The drawing under review shows one solid part. Ordinate dimensions are in mm from its lowest x, y, z. Coordinates: 2 decimals unless noted, no trailing zeros. Write each loop counter-clockwise with the first axis right and the second up, starting at its lowest first coordinate (ties: lowest second). Pieces come first, ordered by that corner, then holes.
Q1. Add section A-A, the plane z = 1188.5. Give the boundary of the cut face in (x, y).
Q2. Add section D-D, the plane x = 1858.5. Give the boundary of the cut face in (y, z) (1 decimal).
Q3. Clearance check with flat-ended pins moving along their axes: pin 1 Ø4 at (y, z) = (9, 1035) entering from -X; pin 2 Ø1.5 at (x, y) = (514, 6.5) entering from -Z; pin 3 Ø12 at (y, z) = (10, 1261.5) entering from -X (1 decimal). State where each tip first meets the part, or that it passes through.
Q4. Add section C-C, the plane z = 457. Give the boundary of the cut face in (x, y).
Q5. To check wall thickness, follow probe 1 along Z at (x, y) = (998.5, 18); probe 2 along Z at (x, y) = (1353, 17.25) (1 decimal); probe 3 along X at (y, z) = (21.25, 431.5) (1 decimal). State the ranges of each line that lie inside material, in increasing order.
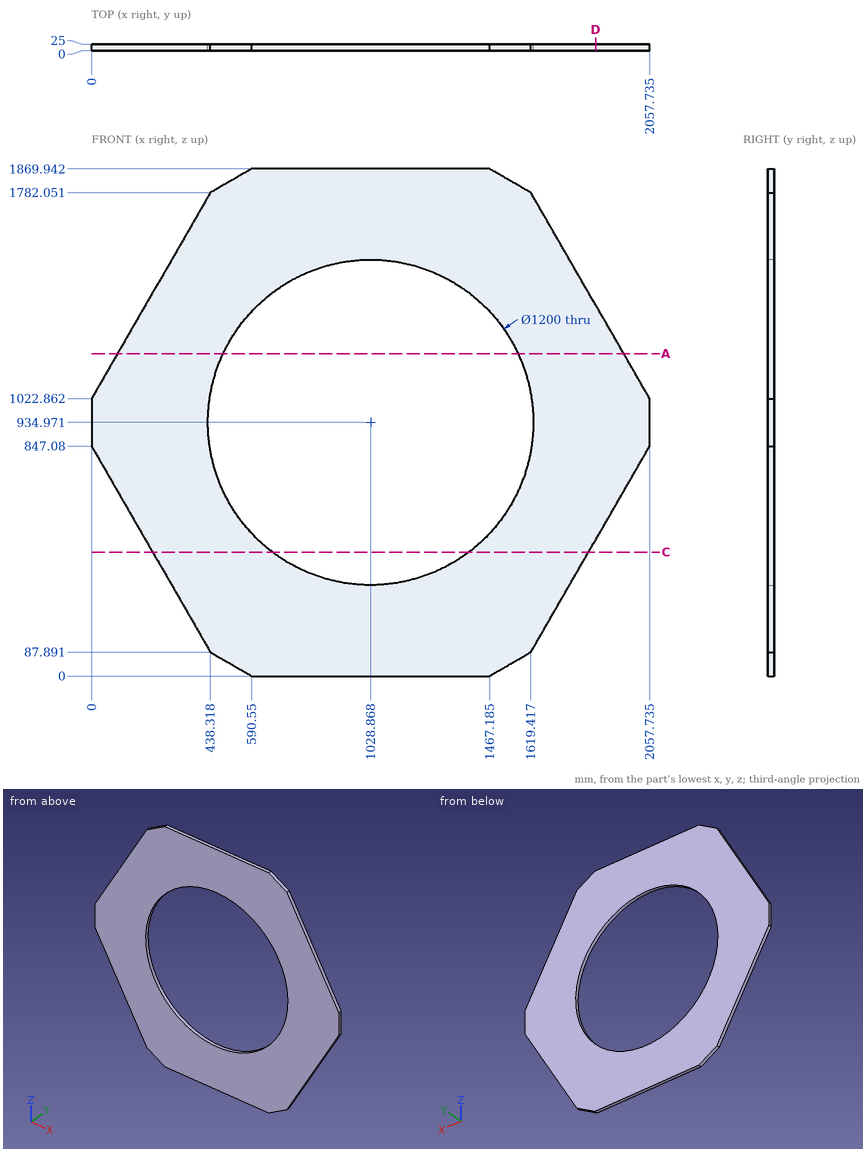
Here are the results:
1. outline: (95.63, 0) - (485.06, 0) - (485.06, 25) - (95.63, 25) - close; (1572.67, 0) - (1962.1, 0) - (1962.1, 25) - (1572.67, 25) - close
2. outline: (0, 502) - (25, 502) - (25, 1367.9) - (0, 1367.9) - close
3. pin 1: stops at x = 5.85
3. pin 2: stops at z = 43.76
3. pin 3: stops at x = 134.3
4. outline: (225.21, 0) - (666.18, 0) - (666.18, 25) - (225.21, 25) - close; (1391.56, 0) - (1832.52, 0) - (1832.52, 25) - (1391.56, 25) - close
5. probe 1: z = 0 to 335.74, 1534.2 to 1869.94
5. probe 2: z = 0 to 430.1, 1439.9 to 1869.9
5. probe 3: x = 239.9 to 702.5, 1355.2 to 1817.8
